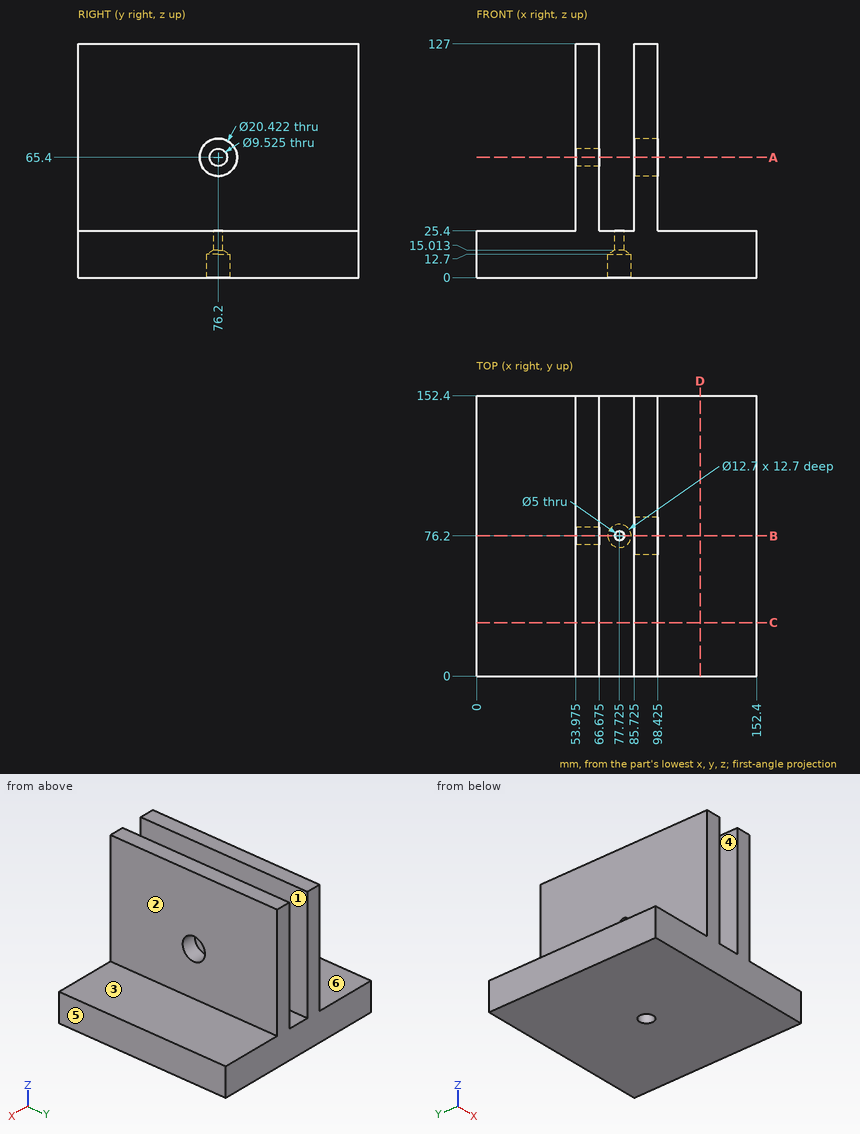
Geometry check sheet. Reference: drawing and pictorial views, mm from the part's lowest x, y, z. A direction names the side the tool comes from. Round coordinates to 2 decimals unless told otherwise and drop trailing zeros. Loops run counter-clockwise (first coordinate to the right, second up) from the corner with the lowest first, then second, coordinate; pieces in that order, holes last. Notation, with made-up numbers: (20.5, -15.75) -> (64.5, -15.75) arc R21 cw to (64.5, 0.25) -> close; hole circle Ø7 at (42.5, 26.5). An arc over 180 degrees is marked (long way). Answer as a JSON object with one key per item and string values.
Q1. Draft check along X on the marked faces 1, 2 and 3. Enter one of: pulls with the +X half, pulls with the -X half, needs draft (parallel to the pull), parting line crosses it, or undercut.
Data:
{"face 1": "undercut", "face 2": "pulls with the +X half", "face 3": "needs draft"}
Q2. Go/stop test with flat-tipped pins: P1, Ø11, axis at y = 76.2, z = 65.4, coming from the -X side (3 decimals); P2, Ø10, axis at x = 32.5, y = 136.5, coming from the +Z side; P3, Ø6, axis at x = 77.725, y = 76.2, coming from the -Z side. Record where each tip stops, or that it passes through.
Data:
{"P1": "stops at x = 53.975", "P2": "stops at z = 25.4", "P3": "stops at z = 14.71"}
Q3. Section check D-D (x = 121.5). Record the boundary of the cut face in (y, z).
Data:
{"outline": "(0, 0) -> (152.4, 0) -> (152.4, 25.4) -> (0, 25.4) -> close"}
Q4. Section check A-A (z = 65.4). Record the boundary of the cut face in (x, y) (1 decimal).
Data:
{"outline": "(54, 0) -> (66.7, 0) -> (66.7, 71.4) -> (54, 71.4) -> close; (54, 81) -> (66.7, 81) -> (66.7, 152.4) -> (54, 152.4) -> close; (85.7, 0) -> (98.4, 0) -> (98.4, 66) -> (85.7, 66) -> close; (85.7, 86.4) -> (98.4, 86.4) -> (98.4, 152.4) -> (85.7, 152.4) -> close"}
Q5. Section check B-B (y = 76.2). Record the boundary of the cut face in (x, z) (1 decimal), then the cut area to 3 significant figures.
Data:
{"outline": "(0, 0) -> (71.4, 0) -> (71.4, 12.7) -> (75.2, 15) -> (75.2, 25.4) -> (66.7, 25.4) -> (66.7, 60.6) -> (54, 60.6) -> (54, 25.4) -> (0, 25.4) -> close; (54, 70.2) -> (66.7, 70.2) -> (66.7, 127) -> (54, 127) -> close; (80.2, 15) -> (84.1, 12.7) -> (84.1, 0) -> (152.4, 0) -> (152.4, 25.4) -> (98.4, 25.4) -> (98.4, 55.2) -> (85.7, 55.2) -> (85.7, 25.4) -> (80.2, 25.4) -> close; (85.7, 75.6) -> (98.4, 75.6) -> (98.4, 127) -> (85.7, 127) -> close", "area": "5,840 mm2"}
Q6. Scan lines: line 1 (X direction, y = 23, z = 99) (1 decimal); line 2 (Z direction, x = 92, y = 76); line 3 (Z direction, x = 60, y = 76). Record each from-to range of solid material in increasing order. Write a range as from..to.
Data:
{"line 1": "x = 54..66.7, 85.7..98.4", "line 2": "z = 0..55.19, 75.61..127", "line 3": "z = 0..60.64, 70.16..127"}
Q7. Section check C-C (y = 29). Record the boundary of the cut face in (x, z) (1 decimal).
Data:
{"outline": "(0, 0) -> (152.4, 0) -> (152.4, 25.4) -> (98.4, 25.4) -> (98.4, 127) -> (85.7, 127) -> (85.7, 25.4) -> (66.7, 25.4) -> (66.7, 127) -> (54, 127) -> (54, 25.4) -> (0, 25.4) -> close"}
Q8. Access from +Z, -Z, +X, -X, +Y, -Y to the whole of each face (thin tool, end or side, straight path). Record for the marked faces 4, 5 and 6.
Data:
{"face 4": "+Z, +Y, -Y", "face 5": "+Z, -Z, +X, +Y, -Y", "face 6": "+Z, -X, +Y, -Y"}
